Here's how the part is built. I have some questions about the finished solid (model axes, mm). A direction names the side the tool comes from. Give positions to 0.01 mm unless a question says otherwise; leave off trailing zeros. Loops run counter-clockwise (first coordinate to the right, second up) from the corner with the lowest first, then second, coordinate; pieces in that order, holes last. Notation, with made-up numbers: (40.25, -18.5) - (91.25, -18.5) arc R20 ccw to (91.25, 12.5) - close; hole circle Ø6 at (-36.75, 51). An arc over 180 degrees is marked (long way). Use one line per item in the form item = value.
from build123d import *

# Parameters (mm, degrees)
SKETCH1_R           = 1.5
SKETCH1_W           = 5
SKETCH1_H           = 5
BOSS_EXTRUDE1_DEPTH = 5
CONG_1_R            = 10


with BuildPart() as part:
    # Sketch1 → Boss-Extrude1 (new body)
    with BuildSketch(Plane.XY):
        Polygon((22.25, 81.5), (22.25, 71.5), (27.25, 71.5), (27.25, 66.5), (22.25, 66.5), (22.25, 63), (19.25, 63), (19.25, 64.1), (16.95, 64.1), (16.95, 63), (12.25, 63), (12.25, 60), (16.95, 60), (16.95, 58.9), (19.25, 58.9), (19.25, 60), (22.25, 60), (22.25, 56.5), (27.25, 56.5), (27.25, 51.5), (22.25, 51.5), (22.25, 31.5), (27.25, 31.5), (27.25, 26.5), (22.25, 26.5), (22.25, 23), (19.25, 23), (19.25, 24.1), (16.95, 24.1), (16.95, 23), (12.25, 23), (12.25, 20), (16.95, 20), (16.95, 18.9), (19.25, 18.9), (19.25, 20), (22.25, 20), (22.25, 16.5), (27.25, 16.5), (27.25, 11.5), (22.25, 11.5), (22.25, 0), (0, 0), (0, 81.5), align=None)
        with Locations((7.5, 47)):
            Circle(SKETCH1_R, mode=Mode.SUBTRACT)
        with Locations((7.5, 17)):
            Circle(SKETCH1_R, mode=Mode.SUBTRACT)
        with Locations((7.5, 39.5)):
            Rectangle(SKETCH1_W, SKETCH1_H, mode=Mode.SUBTRACT)
        with Locations((7.5, 54.5)):
            Rectangle(SKETCH1_W, SKETCH1_H, mode=Mode.SUBTRACT)
        with Locations((7.5, 9.5)):
            Rectangle(SKETCH1_W, SKETCH1_H, mode=Mode.SUBTRACT)
        with Locations((7.5, 24.5)):
            Rectangle(SKETCH1_W, SKETCH1_H, mode=Mode.SUBTRACT)
    extrude(amount=BOSS_EXTRUDE1_DEPTH)

    # Congé1
    cong_1_edges = [part.edges().sort_by_distance(p)[0] for p in [
        (0, 0, 2.5),
        (0, 81.5, 2.5),
    ]]
    fillet(cong_1_edges, radius=CONG_1_R)


solid = part.part
(1) For P1, Ø3, axis at x = 24.5, z = 4, coming from the -Y side; P2, Ø2.5, axis at y = 61, z = 1.5, coming from the +X side; P3, Ø1.5, axis at y = 21.5, z = 3, coming from the +X side, each with a flat end and sliding along its axis, tell me the tip position at first contact or that it passes through.
Geometry says:
P1 = 11.5
P2 = 22.25
P3 = 12.25
(2) If we section it at A-A (x = 15.25): List the corners of the cut face in (y, z) for me.
Geometry says:
outline = (0, 0) - (20, 0) - (20, 5) - (0, 5) - close; (23, 0) - (60, 0) - (60, 5) - (23, 5) - close; (63, 0) - (81.5, 0) - (81.5, 5) - (63, 5) - close
(3) If we section it at D-D (x = 7.5): List the corners of the cut face in (y, z) for me, plus the area to 3 significant figures.
Geometry says:
outline = (0.32, 0) - (7, 0) - (7, 5) - (0.32, 5) - close; (12, 0) - (15.5, 0) - (15.5, 5) - (12, 5) - close; (18.5, 0) - (22, 0) - (22, 5) - (18.5, 5) - close; (27, 0) - (37, 0) - (37, 5) - (27, 5) - close; (42, 0) - (45.5, 0) - (45.5, 5) - (42, 5) - close; (48.5, 0) - (52, 0) - (52, 5) - (48.5, 5) - close; (57, 0) - (81.18, 0) - (81.18, 5) - (57, 5) - close
area = 274 mm²
(4) If we section it at B-B (y = 47): List the corners of the cut face in (x, z) for me.
Geometry says:
outline = (0, 0) - (6, 0) - (6, 5) - (0, 5) - close; (9, 0) - (22.25, 0) - (22.25, 5) - (9, 5) - close
(5) Thinking about a two-plate mould opening in X: for faces 1 (the flat face through (5, 24, 2)), 2 (the cylindrical face through (3.01, 78.65, 2.54)), 3 (the flat face through (22.25, 25, 2)), which applies, pulls with the +X half, pulls with the -X half, needs draft (parallel to the pull), parting line crosses it, or undercut?
Geometry says:
face_1 = undercut
face_2 = pulls with the -X half
face_3 = pulls with the +X half
(6) If I drill on probe 1 along Y at (x, z) = (13.75, 2.5); probe 2 along Y at (x, z) = (23.75, 0.2); probe 3 along Y at (x, z) = (5.5, 3.4), over which ranges is the centre line in solid material (lowest first)?
Geometry says:
probe_1 = 0 to 20, 23 to 60, 63 to 81.5
probe_2 = 11.5 to 16.5, 26.5 to 31.5, 51.5 to 56.5, 66.5 to 71.5
probe_3 = 1.07 to 7, 12 to 22, 27 to 37, 42 to 52, 57 to 80.43
(7) If we section it at C-C (z = 1.9): Give the number of separate pieces and of enclosed holes in the cut face, plus the area to 3 significant figures.
Geometry says:
separate_pieces = 1
enclosed_holes = 6
area = 1,690 mm²
(8) For faces 4 (the flat face through (0, 40, 2)), 5 (the flat face through (25, 11.5, 2)), 6 (the flat face through (7, 7, 2)), which set-ups out of +Z, -Z, +X, -X, +Y, -Y let a thin tool reach every point of the face, with its end or its side?
Geometry says:
face_4 = +Z, -Z, -X, +Y, -Y
face_5 = +Z, -Z, +X, -Y
face_6 = +Z, -Z
